Geometry check sheet. Reference: the model listing, model coordinates, mm. Face numbers are marked on the shaded views. Round coordinates to 2 decimals unless told otherwise and drop trailing zeros. Write each loop counter-clockwise with the first axis right and the second up, starting at its lowest first coordinate (ties: lowest second). Pieces come first, ordered by that corner, then holes. Notation, with made-up numbers: M 12,-7 L 22,-7 A17 cw 22,25 Z; hole C 10,48 d6. An arc over 180 degrees is marked long. Use a Markdown table: item, result.
```python
from build123d import *
from build123d.topology import SkipClean

# Parameters (mm, degrees)
SKETCH1_R                 = 173.85
SKETCH1_R_2               = 131.85
SKETCH1_R_3               = 4.1
BOSS_EXTRUDE1_DEPTH       = 5
BOSS_EXTRUDE2_OUTLINE_R   = 146.85
BOSS_EXTRUDE2_OUTLINE_R_2 = 2.1
BOSS_EXTRUDE2_DEPTH       = 30
CUT_EXTRUDE1_START        = 9.5
SKETCH1_4_R               = 146.85
SKETCH1_4_R_2             = 144.85
CUT_EXTRUDE1_DEPTH        = 2.5
CUT_EXTRUDE2_START        = 21.5
SKETCH1_5_R               = 146.85
SKETCH1_5_R_2             = 144.85
CUT_EXTRUDE2_DEPTH        = 2.5


# Read off the part's stored shape, not the designer's step: Boss-Extrude2
with BuildPart() as part:
    # Sketch1 → Boss-Extrude1 (new body)
    with BuildSketch(Plane(origin=(0, 0, 0), x_dir=(1, 0, 0), z_dir=(0, 1, 0))):
        with Locations(Location((0, 0, 0), (0, 0, 270))):
            Circle(SKETCH1_R)
        with Locations(Location((0, 0, 0), (0, 0, 270))):
            Circle(SKETCH1_R_2, mode=Mode.SUBTRACT)
        with Locations(Location((0, 161.925, 0), (0, 0, 270))):
            Circle(SKETCH1_R_3, mode=Mode.SUBTRACT)
        with Locations(Location((140.231163508, 80.9625, 0), (0, 0, 270))):
            Circle(SKETCH1_R_3, mode=Mode.SUBTRACT)
        with Locations(Location((140.231163508, -80.9625, 0), (0, 0, 270))):
            Circle(SKETCH1_R_3, mode=Mode.SUBTRACT)
        with Locations(Location((0, -161.925, 0), (0, 0, 270))):
            Circle(SKETCH1_R_3, mode=Mode.SUBTRACT)
        with Locations(Location((-140.231163508, -80.9625, 0), (0, 0, 270))):
            Circle(SKETCH1_R_3, mode=Mode.SUBTRACT)
        with Locations(Location((-140.231163508, 80.9625, 0), (0, 0, 270))):
            Circle(SKETCH1_R_3, mode=Mode.SUBTRACT)
    extrude(amount=BOSS_EXTRUDE1_DEPTH)

    # Boss-Extrude2 outline → Boss-Extrude2 (add)
    with BuildSketch(Plane(origin=(0, 0, 0), x_dir=(1, 0, 0), z_dir=(0, 1, 0))):
        Circle(BOSS_EXTRUDE2_OUTLINE_R)
        with Locations((-117.516222284, -55)):
            Circle(BOSS_EXTRUDE2_OUTLINE_R_2, mode=Mode.SUBTRACT)
        with Locations((117.516222284, -55)):
            Circle(BOSS_EXTRUDE2_OUTLINE_R_2, mode=Mode.SUBTRACT)
        with Locations((-117.516222284, 55)):
            Circle(BOSS_EXTRUDE2_OUTLINE_R_2, mode=Mode.SUBTRACT)
        with BuildLine():
            ThreePointArc((-116.687446985, -49.967790594), (-121.499509165, -47.753398598), (-124.505351616, -43.391703343))
            ThreePointArc((-124.505351616, -43.391703343), (-131.85, 0), (-124.505351616, 43.391703343))
            ThreePointArc((-124.505351616, 43.391703343), (-121.499509165, 47.753398598), (-116.687446985, 49.967790594))
            ThreePointArc((-116.687446985, 49.967790594), (-112.897087536, 52.838150289), (-113.121306631, 57.587415004))
            ThreePointArc((-113.121306631, 57.587415004), (-114.503744228, 62.700959824), (-113.080257044, 67.803229768))
            ThreePointArc((-113.080257044, 67.803229768), (0, 131.85), (113.080257044, 67.803229768))
            ThreePointArc((113.080257044, 67.803229768), (114.503744228, 62.700959824), (113.121306631, 57.587415004))
            ThreePointArc((113.121306631, 57.587415004), (112.897087536, 52.838150289), (116.687446985, 49.967790594))
            ThreePointArc((116.687446985, 49.967790594), (121.499509165, 47.753398598), (124.505351616, 43.391703343))
            ThreePointArc((124.505351616, 43.391703343), (131.85, 0), (124.505351616, -43.391703343))
            ThreePointArc((124.505351616, -43.391703343), (121.499509165, -47.753398598), (116.687446985, -49.967790594))
            ThreePointArc((116.687446985, -49.967790594), (112.897087536, -52.838150289), (113.121306631, -57.587415004))
            ThreePointArc((113.121306631, -57.587415004), (114.503744228, -62.700959824), (113.080257044, -67.803229768))
            ThreePointArc((113.080257044, -67.803229768), (0, -131.85), (-113.080257044, -67.803229768))
            ThreePointArc((-113.080257044, -67.803229768), (-114.503744228, -62.700959824), (-113.121306631, -57.587415004))
            ThreePointArc((-113.121306631, -57.587415004), (-112.897087536, -52.838150289), (-116.687446985, -49.967790594))
        make_face(mode=Mode.SUBTRACT)
        with Locations((117.516222284, 55)):
            Circle(BOSS_EXTRUDE2_OUTLINE_R_2, mode=Mode.SUBTRACT)
    extrude(amount=BOSS_EXTRUDE2_DEPTH)

    # Sketch1_4 → Cut-Extrude1 (cut)
    with SkipClean():  # the faces are left unmerged after this step: merging them gives an invalid solid
        with BuildSketch(Plane(origin=(0, 0, 0), x_dir=(1, 0, 0), z_dir=(0, 1, 0)).offset(CUT_EXTRUDE1_START)):
            with Locations(Location((0, 0, 0), (0, 0, 270))):
                Circle(SKETCH1_4_R)
            with Locations(Location((0, 0, 0), (0, 0, 270))):
                Circle(SKETCH1_4_R_2, mode=Mode.SUBTRACT)
        extrude(amount=CUT_EXTRUDE1_DEPTH, mode=Mode.SUBTRACT)

    # Sketch1_5 → Cut-Extrude2 (cut)
    with SkipClean():  # the faces are left unmerged after this step: merging them gives an invalid solid
        with BuildSketch(Plane(origin=(0, 0, 0), x_dir=(1, 0, 0), z_dir=(0, 1, 0)).offset(CUT_EXTRUDE2_START)):
            with Locations(Location((0, 0, 0), (0, 0, 270))):
                Circle(SKETCH1_5_R)
            with Locations(Location((0, 0, 0), (0, 0, 270))):
                Circle(SKETCH1_5_R_2, mode=Mode.SUBTRACT)
        extrude(amount=CUT_EXTRUDE2_DEPTH, mode=Mode.SUBTRACT)


solid = part.part
```
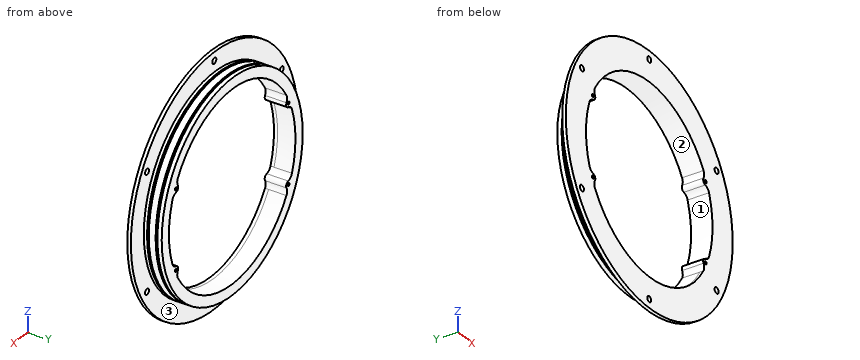
Item 1: Go/stop test with flat-tipped pins: pin 1 (6 mm diameter, centred on y = 14.5, z = 29, fed in from -X); pin 2 (9.5 mm diameter, centred on x = -140.23, z = 80.96, fed in from +Y); pin 3 (4 mm diameter, centred on x = -117.52, z = 55, fed in from -Y); pin 4 (3 mm diameter, centred on y = 7, z = -8.5, fed in from -X). Record where each tip stops, or that it passes through.
Outcome:
| item | result |
|---|---|
| pin 1 | stops at x = -144.53 |
| pin 2 | stops at y = 5 |
| pin 3 | passes through |
| pin 4 | stops at x = -146.68 |
Item 2: Mould release check, pull along X, two halves, no side actions. Record for the marked faces 1, 2 and 3: +X half, -X half, draft (parallel to the pull), parting line (faces both ways), or undercut.
Outcome:
| item | result |
|---|---|
| face 1 | undercut |
| face 2 | undercut |
| face 3 | draft |
Item 3: Cross-section at B-B, the plane x = 10. Record the cut outline in (y, z), and give its area (3 significant figures).
Outcome:
| item | result |
|---|---|
| outline | M 0,-173.56 L 5,-173.56 L 5,-146.51 L 9.5,-146.51 L 9.5,-144.5 L 12,-144.5 L 12,-146.51 L 21.5,-146.51 L 21.5,-144.5 L 24,-144.5 L 24,-146.51 L 30,-146.51 L 30,-131.47 L 0,-131.47 Z; M 0,131.47 L 30,131.47 L 30,146.51 L 24,146.51 L 24,144.5 L 21.5,144.5 L 21.5,146.51 L 12,146.51 L 12,144.5 L 9.5,144.5 L 9.5,146.51 L 5,146.51 L 5,173.56 L 0,173.56 Z |
| area | 1,150 mm2 |
Item 4: Cross-section at A-A, the plane z = 0. Record the cut outline in (x, y), and give its area (3 significant figures).
Outcome:
| item | result |
|---|---|
| outline | M -173.85,0 L -131.85,0 L -131.85,30 L -146.85,30 L -146.85,24 L -144.85,24 L -144.85,21.5 L -146.85,21.5 L -146.85,12 L -144.85,12 L -144.85,9.5 L -146.85,9.5 L -146.85,5 L -173.85,5 Z; M 131.85,0 L 173.85,0 L 173.85,5 L 146.85,5 L 146.85,9.5 L 144.85,9.5 L 144.85,12 L 146.85,12 L 146.85,21.5 L 144.85,21.5 L 144.85,24 L 146.85,24 L 146.85,30 L 131.85,30 Z |
| area | 1,150 mm2 |
Item 5: Cross-section at C-C, the plane z = -106. Record the cut outline in (x, y), and give its area (3 significant figures).
Outcome:
| item | result |
|---|---|
| outline | M -137.8,0 L -78.41,0 L -78.41,30 L -101.63,30 L -101.63,24 L -98.72,24 L -98.72,21.5 L -101.63,21.5 L -101.63,12 L -98.72,12 L -98.72,9.5 L -101.63,9.5 L -101.63,5 L -137.8,5 Z; M 78.41,0 L 137.8,0 L 137.8,5 L 101.63,5 L 101.63,9.5 L 98.72,9.5 L 98.72,12 L 101.63,12 L 101.63,21.5 L 98.72,21.5 L 98.72,24 L 101.63,24 L 101.63,30 L 78.41,30 Z |
| area | 1,730 mm2 |
Item 6: Cross-section at D-D, the plane x = -64. Record the cut outline in (y, z).
Outcome:
| item | result |
|---|---|
| outline | M 0,-161.64 L 5,-161.64 L 5,-132.17 L 9.5,-132.17 L 9.5,-129.94 L 12,-129.94 L 12,-132.17 L 21.5,-132.17 L 21.5,-129.94 L 24,-129.94 L 24,-132.17 L 30,-132.17 L 30,-115.28 L 0,-115.28 Z; M 0,115.28 L 30,115.28 L 30,132.17 L 24,132.17 L 24,129.94 L 21.5,129.94 L 21.5,132.17 L 12,132.17 L 12,129.94 L 9.5,129.94 L 9.5,132.17 L 5,132.17 L 5,161.64 L 0,161.64 Z |
Item 7: Material ranges on line 1 along X through (y, z) = (21, 55); line 2 along Z through (x, y) = (-116, 11.5); line 3 along Y through (x, z) = (-30.5, 158), recorded low to high. Write a range as from..to.
Outcome:
| item | result |
|---|---|
| line 1 | x = -136.16..-119.62, -115.42..-112.42, 112.42..115.42, 119.62..136.16 |
| line 2 | z = -86.75..-56.45, -53.55..-50.13, 50.13..53.55, 56.45..86.75 |
| line 3 | y = 0..5 |
